CAD build for the part. Positions are in the model's coordinates, mm. A direction names the side the tool comes from. Round coordinates to 2 decimals unless told otherwise and drop trailing zeros. Loops run counter-clockwise (first coordinate to the right, second up) from the corner with the lowest first, then second, coordinate; pieces in that order, holes last. Notation, with made-up numbers: (82.25, -30.5) -> (107.25, -30.5) arc R23 cw to (107.25, 3.5) -> close; hole circle Ø11 at (71, -9.75). An arc over 180 degrees is marked (long way). Answer as CSV lines item,"result".
Autodesk Inventor part; units mm, degrees
ref_plane "YZ Plane" through (0, 0, 0) normal (1, 0, 0) x (0, 1, 0)
ref_plane "XZ Plane" through (0, 0, 0) normal (0, 1, 0) x (-1, 0, 0)
ref_plane "XY Plane" through (0, 0, 0) normal (0, 0, 1) x (1, 0, 0)
sketch "Sketch1" plane through (0, 0, 0) normal (0, 0, 1) x (1, 0, 0)
  line L0 (0, 0) -> (19.05, 0)
  line L1 (19.05, 0) -> (19.05, -2.3622)
  line L2 (19.05, -2.3622) -> (14.8082, -2.3622)
  line L3 (14.8082, -2.3622) -> (14.8082, -8.7122)
  line L4 (14.8082, -8.7122) -> (0, -8.7122)
  line L5 (0, -8.7122) -> (0, 0)
  dimension "d2" = 19.05
  dimension "d3" = 2.3622
  dimension "d4" = 4.2418
  dimension "d5" = 6.35
revolve "Revolution1" add sketch "Sketch1" angle 360 about axis through (0, -8.7122, 0) along (0, 1, 0)
sketch "Sketch2" plane through (0, 0, 0) normal (0, 1, 0) x (1, 0, 0)
  circle A0 centre (0, 0) radius 12.5
  dimension "d7" = 25
extrude "Extrusion1" cut sketch "Sketch2" against normal blind 25.4
sketch "Sketch3" plane through (0, -8.7122, 0) normal (0, -1, 0) x (1, 0, 0)
  circle A0 centre (0, 0) radius 14.2875
  circle A1 centre (0, 0) radius 14.8082
  dimension "d10" = 28.575
extrude "Extrusion2" cut sketch "Sketch3" against normal blind 6.35
properties part number "BevelWheelSpace" material "ABS Plastic"
Q1. Slice it at D-D, the plane z = -13. Give the cut face in (x, y), and give its area (3 significant figures).
Results:
outline,"(-13.92, -2.36) -> (-5.93, -2.36) -> (-5.93, -8.71) -> (5.93, -8.71) -> (5.93, -2.36) -> (13.92, -2.36) -> (13.92, 0) -> (-13.92, 0) -> close"
area,"141 mm2"
Q2. Slice it at A-A, the plane z = 0. Give the cut face in (x, y).
Results:
outline,"(-19.05, -2.36) -> (-14.29, -2.36) -> (-14.29, -8.71) -> (-12.5, -8.71) -> (-12.5, 0) -> (-19.05, 0) -> close; (12.5, -8.71) -> (14.29, -8.71) -> (14.29, -2.36) -> (19.05, -2.36) -> (19.05, 0) -> (12.5, 0) -> close"
Q3. Tool access for faces 1 (the flat face through (12.4, 0, 4)), 2 (the cylindrical face through (-14.274, -5.582, 0.628)): list every direction of +Z, -Z, +X, -X, +Y, -Y with a clear straight run to the whole face (end or side of a thin tool).
Results:
face 1,"+Z, -Z, +X, -X, +Y"
face 2,"-Y"
Q4. Probe L1, parallel to Z at x = 0, y = -7; L2, parallel to Y at x = -11.5, z = -14; L3, parallel to X at y = -7, z = 10. List the from-to ranges inside material, lowest first. Write a range as [from, to].
Results:
L1,"[-14.29, -12.5], [12.5, 14.29]"
L2,"[-2.36, 0]"
L3,"[-10.2, -7.5], [7.5, 10.2]"
Q5. Drop flat-ended pins along their axis: pin 1 Ø5 at (y, z) = (-1.5, 5) entering from -X; pin 2 Ø2 at (x, y) = (-6.5, -8) entering from -Z; pin 3 Ø1 at (x, z) = (-11.5, -14) entering from +Y. Give the stop position or say it passes through.
Results:
pin 1,"x = -18.89"
pin 2,"z = -13.19"
pin 3,"y = 0"
Q6. Two-plate mould, pull along X, no slides. Class faces 3 (the flat face through (2.7, -2.362, -14.2)), 4 (the cylindrical face through (11.923, -4.295, -3.755)), 5 (the cylindrical face through (-15.12, -1.2, -11.59)): pulls with the +X half, pulls with the -X half, needs draft (parallel to the pull), parting line crosses it, or undercut.
Results:
face 3,"needs draft"
face 4,"undercut"
face 5,"parting line crosses it"
Q7. Slice it at C-C, the plane y = -7. Give the cut face in (x, z) (1 decimal).
Results:
outline,"circle Ø28.6 at (0, 0); hole circle Ø25 at (0, 0)"
Q8. Slice it at B-B, the plane x = 0. Give the cut face in (y, z).
Results:
outline,"(-8.71, -14.29) -> (-2.36, -14.29) -> (-2.36, -19.05) -> (0, -19.05) -> (0, -12.5) -> (-8.71, -12.5) -> close; (-8.71, 12.5) -> (0, 12.5) -> (0, 19.05) -> (-2.36, 19.05) -> (-2.36, 14.29) -> (-8.71, 14.29) -> close"
